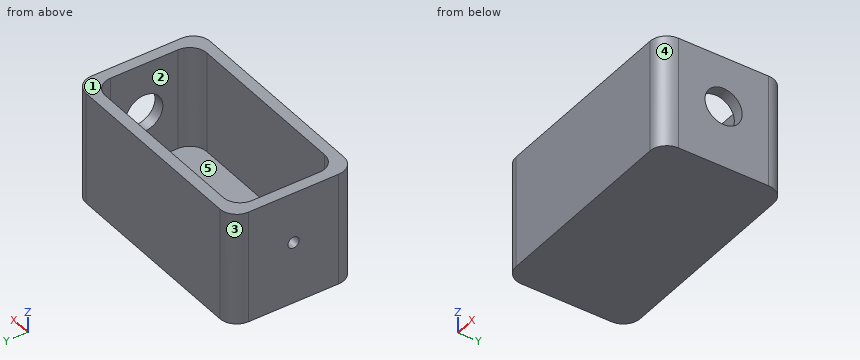
```python
from build123d import *

# Parameters (mm, degrees)
F0_W     = 50.8
F0_H     = 27.94
F1_DEPTH = 25.4
F2_W     = 45.72
F2_H     = 22.86
F3_DEPTH = 22.86
F4_R     = 3.81
F5_R     = 4.191
F6_DEPTH = 2.54
F7_R     = 1.27
F8_DEPTH = 2.54


with BuildPart() as f1:
    # F0 (on Top) → F1 (new body)
    with BuildSketch(Plane.XY):
        Rectangle(F0_W, F0_H)
    extrude(amount=F1_DEPTH)

    # F2 (on face) → F3 (cut)
    with BuildSketch(Plane.XY.offset(25.4)):
        Rectangle(F2_W, F2_H)
    extrude(amount=-F3_DEPTH, mode=Mode.SUBTRACT)

    # F4
    f4_edges = [f1.edges().sort_by_distance(p)[0] for p in [
        (-25.4, -13.97, 12.7),
        (25.4, -13.97, 12.7),
        (25.4, 13.97, 12.7),
        (-25.4, 13.97, 12.7),
        (-22.86, -11.43, 13.97),
        (-22.86, 11.43, 13.97),
        (22.86, 11.43, 13.97),
        (22.86, -11.43, 13.97),
    ]]
    fillet(f4_edges, radius=F4_R)

    # F5 (on face) → F6 (cut, through all)
    with BuildSketch(Plane.YZ.offset(25.4)):
        with Locations((0, 13.97)):
            Circle(F5_R)
    extrude(amount=-F6_DEPTH, mode=Mode.SUBTRACT)

    # F7 (on face) → F8 (cut, through all)
    with BuildSketch(Plane(origin=(-25.4, 0, 0), x_dir=(0, -1, 0), z_dir=(-1, 0, 0))):
        with Locations((0, 13.97)):
            Circle(F7_R)
    extrude(amount=-F8_DEPTH, mode=Mode.SUBTRACT)


solid = f1.part
```
Design review of the part built by this model. Coordinates are the model's own, in mm. Face numbers are marked on the shaded views. A direction names the side the tool comes from. Coordinates: 2 decimals unless noted, no trailing zeros. Loops run counter-clockwise (first coordinate to the right, second up) from the corner with the lowest first, then second, coordinate; pieces in that order, holes last.
Q1. The part is to be moulded in two halves that separate along X. For the marked faces 1, 2 and 3, say which applies: +X half, -X half, draft (parallel to the pull), parting line (faces both ways), or undercut.
Reported:
face 1: draft
face 2: undercut
face 3: -X half
Q2. We need section B-B on y = 0. State the section outline as (x, z) points.
Reported:
outline: (-25.4, 0) - (25.4, 0) - (25.4, 9.78) - (22.86, 9.78) - (22.86, 2.54) - (-22.86, 2.54) - (-22.86, 12.7) - (-25.4, 12.7) - close; (-25.4, 15.24) - (-22.86, 15.24) - (-22.86, 25.4) - (-25.4, 25.4) - close; (22.86, 18.16) - (25.4, 18.16) - (25.4, 25.4) - (22.86, 25.4) - close
Q3. For pin 1 (2 mm diameter, centred on y = 0, z = 13.97, fed in from +X) (1 decimal), flat-tipped, find the tip position at first contact; note if it passes through.
Reported:
pin 1: passes through
Q4. We need section D-D on z = 4.25. State the section outline as (x, y) points.
Reported:
outline: (-25.4, -10.16) arc R3.81 ccw to (-21.59, -13.97) - (21.59, -13.97) arc R3.81 ccw to (25.4, -10.16) - (25.4, 10.16) arc R3.81 ccw to (21.59, 13.97) - (-21.59, 13.97) arc R3.81 ccw to (-25.4, 10.16) - close; hole (-22.86, -7.62) arc R3.81 ccw to (-19.05, -11.43) - (19.05, -11.43) arc R3.81 ccw to (22.86, -7.62) - (22.86, 7.62) arc R3.81 ccw to (19.05, 11.43) - (-19.05, 11.43) arc R3.81 ccw to (-22.86, 7.62) - close
Q5. To check wall thickness, follow line 1 (Y direction, x = 16, z = 2.75); line 2 (X direction, y = -2.25, z = 18); line 3 (Z direction, x = 24.75, y = 0). State the ranges of each line that lie inside material, in increasing order.
Reported:
line 1: y = -13.97 to -11.43, 11.43 to 13.97
line 2: x = -25.4 to -22.86, 22.86 to 25.4
line 3: z = 0 to 9.78, 18.16 to 25.4
Q6. Tool access review of the marked faces 4 and 5: name each direction out of +Z, -Z, +X, -X, +Y, -Y from which nothing blocks a thin tool from reaching the whole face with its end or side.
Reported:
face 4: +Z, -Z, +X, -Y
face 5: +Z
Q7. We need section A-A on z = 13.97. State the section outline as (x, y) points.
Reported:
outline: (-25.4, -10.16) arc R3.81 ccw to (-21.59, -13.97) - (21.59, -13.97) arc R3.81 ccw to (25.4, -10.16) - (25.4, -4.19) - (22.86, -4.19) - (22.86, -7.62) arc R3.81 cw to (19.05, -11.43) - (-19.05, -11.43) arc R3.81 cw to (-22.86, -7.62) - (-22.86, -1.27) - (-25.4, -1.27) - close; (-25.4, 1.27) - (-22.86, 1.27) - (-22.86, 7.62) arc R3.81 cw to (-19.05, 11.43) - (19.05, 11.43) arc R3.81 cw to (22.86, 7.62) - (22.86, 4.19) - (25.4, 4.19) - (25.4, 10.16) arc R3.81 ccw to (21.59, 13.97) - (-21.59, 13.97) arc R3.81 ccw to (-25.4, 10.16) - close
Q8. We need section C-C on x = -11. State the section outline as (y, z) points.
Reported:
outline: (-13.97, 0) - (13.97, 0) - (13.97, 25.4) - (11.43, 25.4) - (11.43, 2.54) - (-11.43, 2.54) - (-11.43, 25.4) - (-13.97, 25.4) - close
